Check sheet for the modelled part. Datum: model origin and axes. Units: mm. A direction names the side the tool comes from. Round coordinates to 2 decimals unless told otherwise and drop trailing zeros. Order: outer loops, then holes, each group sorted by start corner. A loop starts at its lowest first (then second) coordinate and runs counter-clockwise, first axis right, second up.
Q1. Depth check by flat-ended pin: P1, Ø11.5, axis at x = 0, z = 0, coming from the -Y side; P2, Ø3, axis at x = 3.5, y = 2, coming from the -Z side; P3, Ø1.5, axis at x = -16.5, z = -25, coming from the +Y side. Enter the tip coordinate at first touch or a pass-through.
Q2. Cross-section at C-C on y = 1.1. Record the cut outline in (x, z).
Q3. Scan lines: probe 1 along X at (y, z) = (3.45, 0); probe 2 along Y at (x, z) = (11.5, -20.5); probe 3 along Z at (x, y) = (12, 3.75). Record each from-to range of solid material in increasing order.
Q4. Cross-section at B-B on x = 0. Record the cut outline in (y, z).
Q5. Cross-section at D-D on z = -14.5. Record the cut outline in (x, y), then the cut area to 3 significant figures.
Q6. Cross-section at A-A on z = 0. Record the cut outline in (x, y), then the cut area to 3 significant figures.
Q7. Set-up check for faces 4 (the cylindrical face through (-0.267, 1.014, -24.537)), 5 (the cylindrical face through (-22, -1, 0)), 6 (the flat face through (1, 2, 9)): record each of +Z, -Z, +X, -X, +Y, -Y from which the full face is reachable in a straight line by a thin tool's end or side.
Q8. Mould release check, pull along X, two halves, no side actions. Record for faces 1 (the flat face through (20, -2, 0)), 2 (the cylindrical face through (-39.05, 1.97, -8.67)), 3 (the cylindrical face through (18, -1, 0)): +X half, -X half, draft (parallel to the pull), parting line (faces both ways), or undercut.
from build123d import *

# Parameters (mm, degrees)
SKETCH1_R           = 40
BOSS_EXTRUDE1_DEPTH = 40
SKETCH2_R           = 38
CUT_EXTRUDE1_DEPTH  = 38
CUT_EXTRUDE2_DEPTH  = 38
SKETCH4_R           = 5
CUT_EXTRUDE3_DEPTH  = 38
SKETCH6_R           = 2
BOSS_EXTRUDE2_DEPTH = 2
SKETCH8_R           = 43.496918112
CUT_EXTRUDE4_DEPTH  = 36


with BuildPart() as part:
    # Sketch1 → Boss-Extrude1 (new body)
    with BuildSketch(Plane(origin=(0, 0, 0), x_dir=(1, 0, 0), z_dir=(0, 1, 0))):
        with Locations(Location((0, 0, 0), (0, 0, 270))):
            Circle(SKETCH1_R)
    extrude(amount=BOSS_EXTRUDE1_DEPTH)

    # Sketch2 → Cut-Extrude1 (cut)
    with BuildSketch(Plane(origin=(0, 40, 0), x_dir=(1, 0, 0), z_dir=(0, 1, 0))):
        with Locations(Location((0, 0, 0), (0, 0, 270))):
            Circle(SKETCH2_R)
    extrude(amount=-CUT_EXTRUDE1_DEPTH, mode=Mode.SUBTRACT)

    # Sketch3 → Cut-Extrude2 (cut)
    with BuildSketch(Plane(origin=(0, 2, 0), x_dir=(1, 0, 0), z_dir=(0, 1, 0))):
        with BuildLine():
            ThreePointArc((-14.076066703, 35.296803626), (0, 24.534862453), (14.076066703, 35.296803626))
            ThreePointArc((14.076066703, 35.296803626), (0, 38), (-14.076066703, 35.296803626))
        make_face()
    extrude(amount=-CUT_EXTRUDE2_DEPTH, mode=Mode.SUBTRACT)

    # Sketch4 → Cut-Extrude3 (cut)
    with BuildSketch(Plane(origin=(0, 2, 0), x_dir=(1, 0, 0), z_dir=(0, 1, 0))):
        with Locations(Location((0, 0, 0), (0, 0, 270))):
            Circle(SKETCH4_R)
    extrude(amount=-CUT_EXTRUDE3_DEPTH, mode=Mode.SUBTRACT)

    # Sketch6 → Boss-Extrude2 (add)
    with BuildSketch(Plane.XZ):
        with Locations(Location((-20, 0, 0), (0, 0, 90))):
            Circle(SKETCH6_R)
        with Locations(Location((20, 0, 0), (0, 0, 90))):
            Circle(SKETCH6_R)
    extrude(amount=BOSS_EXTRUDE2_DEPTH)

    # Sketch8 → Cut-Extrude4 (cut)
    with BuildSketch(Plane(origin=(0, 40, 0), x_dir=(1, 0, 0), z_dir=(0, 1, 0))):
        Circle(SKETCH8_R)
    extrude(amount=-CUT_EXTRUDE4_DEPTH, mode=Mode.SUBTRACT)


solid = part.part
Results found:
1. P1: stops at y = 0
1. P2: stops at z = -39.95
1. P3: stops at y = 2
2. outline: circle Ø80 at (0, 0); hole (-14.08, -35.3) arc R38 ccw to (14.08, -35.3) arc R14.59 ccw to start; hole circle Ø10 at (0, 0)
3. probe 1: x = -40 to -38, 38 to 40
3. probe 2: y = 0 to 2
3. probe 3: z = -38.16 to -36.06, 36.06 to 38.16
4. outline: (0, -40) - (4, -40) - (4, -38) - (0, -38) - close; (0, -24.53) - (2, -24.53) - (2, -5) - (0, -5) - close; (0, 5) - (2, 5) - (2, 38) - (4, 38) - (4, 40) - (0, 40) - close
5. outline: (-37.28, 0) - (37.28, 0) - (37.28, 4) - (35.12, 4) - (35.12, 2) - (-35.12, 2) - (-35.12, 4) - (-37.28, 4) - close
5. area: 158 mm2
6. outline: (-40, 0) - (-22, 0) - (-22, -2) - (-18, -2) - (-18, 0) - (-5, 0) - (-5, 2) - (-38, 2) - (-38, 4) - (-40, 4) - close; (5, 0) - (18, 0) - (18, -2) - (22, -2) - (22, 0) - (40, 0) - (40, 4) - (38, 4) - (38, 2) - (5, 2) - close
6. area: 164 mm2
7. face 4: +Y, -Y
7. face 5: -Y
7. face 6: +Y
8. face 1: draft
8. face 2: parting line
8. face 3: undercut
